Here's how the part is built. I have some questions about the finished solid (model axes, mm). Face numbers are marked on the shaded views. A direction names the side the tool comes from. Coordinates: 2 decimals unless noted, no trailing zeros. Loops run counter-clockwise (first coordinate to the right, second up) from the corner with the lowest first, then second, coordinate; pieces in that order, holes last. Notation, with made-up numbers: (0, -37.5) -> (53, -37.5) arc R28 cw to (53, -11.5) -> close; hole circle Ø2 at (83.25, 49). An arc over 180 degrees is marked (long way). Answer as a JSON object with one key per item and string values. Group by question number.
1) I want a section at A-A (x = 34.5). Write out the boundary of the cut face in (y, z).
2) I want a section at D-D (x = 0). Write out the boundary of the cut face in (y, z) (3 decimals).
3) I'm going to push flat-ended pins straight in: pin 1 (12 mm diameter, centred on x = -1.5, z = 22.5, fed in from +Y); pin 2 (2.5 mm diameter, centred on x = 35, y = 3, fed in from +Z); pin 3 (5 mm diameter, centred on x = 34.5, y = 5, fed in from -Z); pin 4 (1.8 mm diameter, centred on x = -14.5, y = 5, fed in from +Z). Where does each tip first touch, or does it pass through?
4) If we mould it in two halves opening along Z, with no side actions, what happens to the marked faces 1, 2, 3 and 4? For each: +Z half, -Z half, draft (parallel to the pull), parting line (faces both ways), or undercut.
5) Which directions (+Z, -Z, +X, -X, +Y, -Y) give clear straight access to the entire face, cutting with the end or side of a thin tool? Please do the marked faces 5, 6, 7, 8 and 9.
6) I need wall thicknesses on probe 1 along Y at (x, z) = (34.5, 28); probe 2 along X at (y, z) = (-5, 28); probe 3 along Z at (x, y) = (-4.5, 1.25). Which ranges of each line are inside material? Lowest first, please. Write a range as [from, to].
7) I want a section at B-B (y = 8). Write out the boundary of the cut face in (x, z).
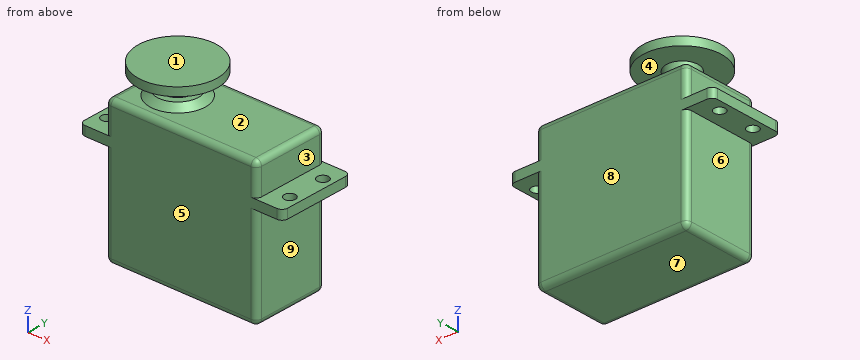
```python
from build123d import *

# Parameters (mm, degrees)
CYLINDER001_R     = 3
CYLINDER001_DEPTH = 4.5
CYLINDER002_R     = 1.5
CYLINDER002_DEPTH = 5
BOX001_W          = 54.5
BOX001_H          = 20.5
BOX001_DEPTH      = 2.5
FILLET_R          = 1.5
FILLET001_R       = 1.5
FILLET002_R       = 1.5
FILLET003_R       = 1.5
BOX_W             = 40.5
BOX_H             = 20.5
BOX_DEPTH         = 38
FILLET004_R       = 1.5
CYLINDER_R        = 10.5
CYLINDER_DEPTH    = 2.25


with BuildPart() as servobodycone:
    # Cone → Cone (revolve)
    with BuildSketch(Plane(origin=(0, 0, 37.5), x_dir=(1, 0, 0), z_dir=(0, -1, 0))):
        Polygon((0, 0), (8, 0), (5.5, 2), (0, 2), align=None)
    revolve(axis=Axis((0, 0, 37.5), (0, 0, 1)))


with BuildPart() as cone001:
    # Cone001 → Cone001 (revolve)
    with BuildSketch(Plane(origin=(0, 0, 39.75), x_dir=(1, 0, 0), z_dir=(0, -1, 0))):
        Polygon((0, 0), (4.12, 0), (4.25, 4), (0, 4), align=None)
    revolve(axis=Axis((0, 0, 39.75), (0, 0, 1)))


with BuildPart() as shaft:
    # Cylinder001 → Cylinder001 (new body)
    with BuildSketch(Plane.XY.offset(38.5)):
        Circle(CYLINDER001_R)
    extrude(amount=CYLINDER001_DEPTH)


with BuildPart() as screw_hole1:
    # Cylinder002 → Cylinder002 (new body)
    with BuildSketch(Plane(origin=(-14.5, 5, 26), x_dir=(1, 0, 0), z_dir=(0, 0, 1))):
        Circle(CYLINDER002_R)
    extrude(amount=CYLINDER002_DEPTH)


with BuildPart() as screw_hole3:
    # Clone001 base: copy of Screw_hole1
    add(screw_hole1.part)


with BuildPart() as screw_hole3_1:
    # Clone001 placement: moved
    add(screw_hole3.part.moved(Location((49, 0, 0))))


with BuildPart() as screw_hole4:
    # Clone002 base: copy of Screw_hole3
    add(screw_hole3_1.part)


with BuildPart() as screw_hole4_1:
    # Clone002 placement: moved
    add(screw_hole4.part.moved(Location((0, -10, 0))))


with BuildPart() as screw_hole2:
    # Clone base: copy of Screw_hole1
    add(screw_hole1.part)


with BuildPart() as screw_hole2_1:
    # Clone placement: moved
    add(screw_hole2.part.moved(Location((0, -10, 0))))


with BuildPart() as servo_lugs001:
    # Box001 → Box001 (new body)
    with BuildSketch(Plane(origin=(-17.25, -10.25, 27), x_dir=(1, 0, 0), z_dir=(0, 0, 1))):
        with Locations((27.25, 10.25)):
            Rectangle(BOX001_W, BOX001_H)
    extrude(amount=BOX001_DEPTH)

    # Cut: cut Screw_hole1
    add(screw_hole1.part, mode=Mode.SUBTRACT)

    # Cut001: cut Screw_hole2
    add(screw_hole2_1.part, mode=Mode.SUBTRACT)

    # Cut002: cut Screw_hole3
    add(screw_hole3_1.part, mode=Mode.SUBTRACT)

    # Cut003: cut Screw_hole4
    add(screw_hole4_1.part, mode=Mode.SUBTRACT)

    # Fillet
    fillet_edges = [servo_lugs001.edges().sort_by_distance(p)[0] for p in [
        (37.25, -10.25, 28.25),
    ]]
    fillet(fillet_edges, radius=FILLET_R)

    # Fillet001
    fillet001_edges = [servo_lugs001.edges().sort_by_distance(p)[0] for p in [
        (37.25, 10.25, 28.25),
    ]]
    fillet(fillet001_edges, radius=FILLET001_R)

    # Fillet002
    fillet002_edges = [servo_lugs001.edges().sort_by_distance(p)[0] for p in [
        (-17.25, -10.25, 28.25),
    ]]
    fillet(fillet002_edges, radius=FILLET002_R)

    # Fillet003
    fillet003_edges = [servo_lugs001.edges().sort_by_distance(p)[0] for p in [
        (-17.25, 10.25, 28.25),
    ]]
    fillet(fillet003_edges, radius=FILLET003_R)


with BuildPart() as servobody001:
    # Box → Box (new body)
    with BuildSketch(Plane(origin=(-10.25, -10.25, 0), x_dir=(1, 0, 0), z_dir=(0, 0, 1))):
        with Locations((20.25, 10.25)):
            Rectangle(BOX_W, BOX_H)
    extrude(amount=BOX_DEPTH)

    # Fillet004
    fillet004_edges = [servobody001.edges().sort_by_distance(p)[0] for p in [
        (-10.25, -10.25, 19),
        (-10.25, 0, 38),
        (-10.25, 10.25, 19),
        (-10.25, 0, 0),
        (30.25, -10.25, 19),
        (30.25, 0, 38),
        (30.25, 10.25, 19),
        (30.25, 0, 0),
        (10, -10.25, 0),
        (10, -10.25, 38),
        (10, 10.25, 0),
        (10, 10.25, 38),
    ]]
    fillet(fillet004_edges, radius=FILLET004_R)


with BuildPart() as servo:
    # Cylinder → Cylinder (new body)
    with BuildSketch(Plane.XY.offset(43.5)):
        Circle(CYLINDER_R)
    extrude(amount=CYLINDER_DEPTH)

    # Fusion: union ServoBodyCone, Cone001, shaft, servo_lugs001, ServoBody001
    add(servobodycone.part)
    add(cone001.part)
    add(shaft.part)
    add(servo_lugs001.part)
    add(servobody001.part)


solid = servo.part
```
Determined:
{
 "1": {"outline": "(-10.25, 27) -> (-6.5, 27) -> (-6.5, 29.5) -> (-10.25, 29.5) -> close; (-3.5, 27) -> (3.5, 27) -> (3.5, 29.5) -> (-3.5, 29.5) -> close; (6.5, 27) -> (10.25, 27) -> (10.25, 29.5) -> (6.5, 29.5) -> close"},
 "2": {"outline": "(-10.5, 43.5) -> (-4.242, 43.5) -> (-4.12, 39.75) -> (-3, 39.75) -> (-3, 39.5) -> (-5.5, 39.5) -> (-7.375, 38) -> (-8.75, 38) arc R1.5 ccw to (-10.25, 36.5) -> (-10.25, 1.5) arc R1.5 ccw to (-8.75, 0) -> (8.75, 0) arc R1.5 ccw to (10.25, 1.5) -> (10.25, 36.5) arc R1.5 ccw to (8.75, 38) -> (7.375, 38) -> (5.5, 39.5) -> (3, 39.5) -> (3, 39.75) -> (4.12, 39.75) -> (4.242, 43.5) -> (10.5, 43.5) -> (10.5, 45.75) -> (-10.5, 45.75) -> close"},
 "3": {"pin 1": "y = 10.25", "pin 2": "z = 29.5", "pin 3": "z = 27", "pin 4": "through"},
 "4": {"face 1": "+Z half", "face 2": "undercut", "face 3": "draft", "face 4": "undercut"},
 "5": {"face 5": "-Z, +X, -X, -Y", "face 6": "-Z, -X, +Y, -Y", "face 7": "-Z, +X, -X, +Y, -Y", "face 8": "-Z, +X, -X, +Y", "face 9": "-Z, +X, +Y, -Y"},
 "6": {"probe 1": "[-10.25, -6.5], [-3.5, 3.5], [6.5, 10.25]", "probe 2": "[-17.25, -16], [-13, 33], [36, 37.25]", "probe 3": "[0, 39.5], [43.5, 45.75]"},
 "7": {"outline": "(-17.25, 27) -> (-10.25, 27) -> (-10.25, 1.5) arc R1.5 ccw to (-8.75, 0) -> (28.75, 0) arc R1.5 ccw to (30.25, 1.5) -> (30.25, 27) -> (37.25, 27) -> (37.25, 29.5) -> (30.25, 29.5) -> (30.25, 36.5) arc R1.5 ccw to (28.75, 38) -> (-8.75, 38) arc R1.5 ccw to (-10.25, 36.5) -> (-10.25, 29.5) -> (-17.25, 29.5) -> close; (-6.8, 43.5) -> (6.8, 43.5) -> (6.8, 45.75) -> (-6.8, 45.75) -> close"}
}
